Autodesk Inventor part; units mm, degrees
ref_plane "YZ Plane" through (0, 0, 0) normal (1, 0, 0) x (0, 1, 0)
ref_plane "XZ Plane" through (0, 0, 0) normal (0, 1, 0) x (-1, 0, 0)
ref_plane "XY Plane" through (0, 0, 0) normal (0, 0, 1) x (1, 0, 0)
sketch "Sketch1" plane through (0, 0, 0) normal (0, 1, 0) x (-1, 0, 0)
  line L0 (-17.018, 36.3476) -> (-17.018, 3.1529)
  line L1 (-15.4305, 0.4033) -> (-8.9535, -3.3362)
  line L2 (-5.7785, -3.3362) -> (0, 0)
  line L3 (-15.4305, 39.0972) -> (-8.9535, 42.8367)
  line L4 (-5.7785, 42.8367) -> (0, 39.5005)
  arc A0 (-15.4305, 39.0972) -> (-17.018, 36.3476) centre (-13.843, 36.3476) ccw
  arc A1 (-5.7785, 42.8367) -> (-8.9535, 42.8367) centre (-7.366, 40.0871) ccw
  arc A2 (-8.9535, -3.3362) -> (-5.7785, -3.3362) centre (-7.366, -0.5866) ccw
  arc A3 (-17.018, 3.1529) -> (-15.4305, 0.4033) centre (-13.843, 3.1529) ccw
  line L5 (-0.635, 1.0999) -> (-6.4135, -2.2364)
  arc A4 (-8.3185, -2.2364) -> (-6.4135, -2.2364) centre (-7.366, -0.5866) ccw
  line L6 (-8.3185, -2.2364) -> (-14.7955, 1.5031)
  arc A5 (-15.748, 3.1529) -> (-14.7955, 1.5031) centre (-13.843, 3.1529) ccw
  line L7 (-15.748, 3.1529) -> (-15.748, 36.3476)
  arc A6 (-14.7955, 37.9973) -> (-15.748, 36.3476) centre (-13.843, 36.3476) ccw
  line L8 (-14.7955, 37.9973) -> (-8.3185, 41.7368)
  arc A7 (-6.4135, 41.7368) -> (-8.3185, 41.7368) centre (-7.366, 40.0871) ccw
  line L9 (-6.4135, 41.7368) -> (-0.635, 38.4006)
  line L10 (0, 39.5005) -> (-0.635, 38.4006)
  line L11 (-0.635, 1.0999) -> (0, 0)
  point P0 (-17.018, 38.1807)
  point P1 (-17.018, 1.3198)
  point P2 (-7.366, -4.2528)
  point P3 (-7.366, 43.7532)
  dimension "d2" = 48.006
  dimension "d3" = 17.018
  dimension "d4" = 17.018
  dimension "d5" = 120
  dimension "d6" = 120
  dimension "d7" = 120
  dimension "d8" = 120
  dimension "d9" = 9.652
  dimension "d10" = 9.652
  dimension "d11" = 3.175
  dimension "d12" = 1.27
extrude "Extrusion1" add sketch "Sketch1" along normal blind 290.068
sketch "Sketch2" plane through (15.748, 0, 3.1529) normal (-1, 0, 0) x (0, 0, 1)
  line L0 (13.0392, 6.096) -> (13.0392, 90.932)
  line L1 (20.1512, 6.096) -> (20.1512, 90.932)
  arc A0 (20.1512, 90.932) -> (13.0392, 90.932) centre (16.5952, 90.932) ccw
  arc A1 (13.0392, 6.096) -> (20.1512, 6.096) centre (16.5952, 6.096) ccw
  line L2 (13.0392, 199.136) -> (13.0392, 283.972)
  line L3 (20.1512, 199.136) -> (20.1512, 283.972)
  arc A2 (20.1512, 283.972) -> (13.0392, 283.972) centre (16.5952, 283.972) ccw
  arc A3 (13.0392, 199.136) -> (20.1512, 199.136) centre (16.5952, 199.136) ccw
  line L4 (0, 0) -> (33.1947, 0)
  line L5 (39.6838, 0) -> (39.6838, 290.068)
  point P0 (-3.1529, 0)
  point P1 (16.5952, 94.488)
  point P2 (16.5952, 2.54)
  point P3 (16.5952, 94.488)
  point P4 (16.5952, 195.58)
  point P5 (16.5952, 287.528)
  dimension "d16" = 101.092
  dimension "d17" = 91.948
  dimension "d18" = 91.948
  dimension "d19" = 2.54
  dimension "d20" = 23.0886
  dimension "d21" = 23.0886
  dimension "d22" = 7.112
  dimension "d23" = 7.112
extrude "Extrusion2" cut sketch "Sketch2" against normal through all
properties part number "PoleBracket"
Geometry: final body of the model. Coordinates: model frame, mm. A direction names the side the tool comes from. Give positions to 0.01 mm unless a question says otherwise; leave off trailing zeros. Loops run counter-clockwise (first coordinate to the right, second up) from the corner with the lowest first, then second, coordinate; pieces in that order, holes last. Notation, with made-up numbers: M 8.25,49.25 L 13.25,49.25 A13 cw 13.25,65.25 Z; hole C 68.5,-1.75 d1. An arc over 180 degrees is marked long. Put each result on its own line as item: value. Start each with the question number.
1) Ray query, line 1 along Z through (x, y) = (7, 221.5); line 2 along X through (y, z) = (48, 6.5); line 3 along Z through (x, y) = (11.25, 236). Return the intervals inside material, ascending.
2) Cut plane A-A (y = 81.5). Output: boundary loops of the cut face in (x, z) (1 decimal).
3) Access query for faces 1 (the flat face through (17.018, 143, 20)), 2 (the flat face through (11.6, 143, 39.84)). Directions: +Z, -Z, +X, -X, +Y, -Y. A direction counts if a zero-diameter tool reaches every point of the face in a straight line with its end or side. Return the directions, or none.
4) Contact query for flat-ended pins moving along their axis: pin 1 (1.4 mm diameter, centred on x = 16, y = 30, fed in from +Z); pin 2 (1 mm diameter, centred on x = 15, y = 230, fed in from +Z); pin 3 (1.5 mm diameter, centred on y = 228, z = 33, fed in from -X); pin 4 (2 mm diameter, centred on x = 13, z = 31.5, fed in from +Y). Output: stop coordinate, or through.
5) Pull-direction query (Z, two-part tool) for faces 3 (the flat face through (12.24, 143, -1.44)), 4 (the flat face through (16, 0, 20)), 5 (the flat face through (15.748, 143, 20)); classes: pulls with the +Z half, pulls with the -Z half, needs draft (parallel to the pull), parting line crosses it, or undercut.
6) Cut plane C-C (z = 27.5). Output: boundary loops of the cut face in (x, y), then the cut area to 3 significant figures.
7) Cut plane B-B (y = 157). Output: boundary loops of the cut face in (x, z) (1 decimal), then the cut area to 3 significant figures.
Verdict:
1. line 1: -3.74 to -2.46, 41.96 to 43.24
1. line 2: 15.75 to 17.02
1. line 3: -2.01 to -0.54, 40.04 to 41.51
2. outline: M 0,0 L 5.8,-3.3 A3.2 ccw 9,-3.3 L 15.4,0.4 A3.2 ccw 17,3.2 L 17,16.2 L 15.7,16.2 L 15.7,3.2 A1.9 cw 14.8,1.5 L 8.3,-2.2 A1.9 cw 6.4,-2.2 L 0.6,1.1 Z; M 0,39.5 L 0.6,38.4 L 6.4,41.7 A1.9 cw 8.3,41.7 L 14.8,38 A1.9 cw 15.7,36.3 L 15.7,23.3 L 17,23.3 L 17,36.3 A3.2 ccw 15.4,39.1 L 9,42.8 A3.2 ccw 5.8,42.8 Z
3. face 1: +Z, -Z, +X, +Y, -Y
3. face 2: +Y, -Y
4. pin 1: z = 39.17
4. pin 2: z = 39.63
4. pin 3: x = 15.75
4. pin 4: through
5. face 3: pulls with the -Z half
5. face 4: needs draft
5. face 5: undercut
6. outline: M 15.75,0 L 17.02,0 L 17.02,290.07 L 15.75,290.07 Z
6. area: 368 mm2
7. outline: M 0,0 L 5.8,-3.3 A3.2 ccw 9,-3.3 L 15.4,0.4 A3.2 ccw 17,3.2 L 17,36.3 A3.2 ccw 15.4,39.1 L 9,42.8 A3.2 ccw 5.8,42.8 L 0,39.5 L 0.6,38.4 L 6.4,41.7 A1.9 cw 8.3,41.7 L 14.8,38 A1.9 cw 15.7,36.3 L 15.7,3.2 A1.9 cw 14.8,1.5 L 8.3,-2.2 A1.9 cw 6.4,-2.2 L 0.6,1.1 Z
7. area: 91.6 mm2
